Geometry: see drawing. Coordinates: mm, zero at the bounding-box minimum. Round coordinates to 2 decimals unless told otherwise and drop trailing zeros. Loops run counter-clockwise (first coordinate to the right, second up) from the corner with the lowest first, then second, coordinate; pieces in that order, holes last.
(1) Section C-C, the plane y = 1.4. Return the cut outline in (x, z).
(2) Mould query, pull axis Z, two halves, no side actions, for the marked faces 1, 2 and 3. Classes: pulls with the +Z half, pulls with the -Z half, needs draft (parallel to the pull), parting line crosses it, or undercut.
(3) Section B-B, the plane z = 26.67. Return the cut outline in (x, y), plus the area to 3 significant figures.
(4) Section D-D, the plane x = 42. Return the cut outline in (y, z), plus the area to 3 significant figures.
(5) Material intervals for probe 1 along Z at (x, y) = (26.67, 3.4); probe 2 along X at (y, z) = (2.3, 45.72); probe 3 along Z at (x, y) = (31.5, 1.6), sorted ascending.
(6) First-contact query: pin 1 Ø3 at (x, y) = (11.5, 4) entering from +Z; pin 2 Ø1.5 at (x, y) = (12.5, 3.5) entering from -Z; pin 3 Ø2.5 at (x, y) = (27, 3) entering from -Z. Flat tips, straight axial feed; report the tip coordinate or a pass-through.
(7) Section A-A, the plane x = 26.67. Return the cut outline in (y, z).
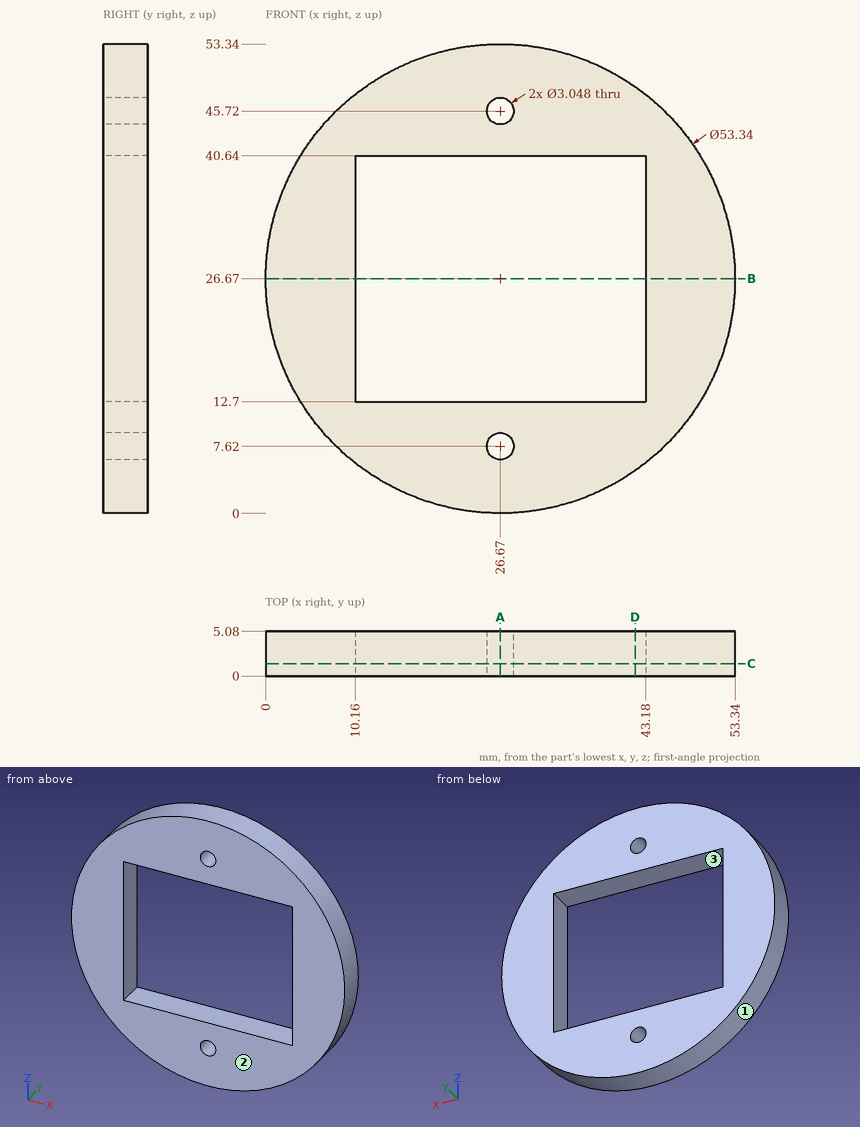
Output values:
1. outline: circle Ø53.34 at (26.67, 26.67); hole (10.16, 12.7) - (43.18, 12.7) - (43.18, 40.64) - (10.16, 40.64) - close; hole circle Ø3.05 at (26.67, 7.62); hole circle Ø3.05 at (26.67, 45.72)
2. face 1: parting line crosses it
2. face 2: needs draft
2. face 3: undercut
3. outline: (0, 0) - (10.16, 0) - (10.16, 5.08) - (0, 5.08) - close; (43.18, 0) - (53.34, 0) - (53.34, 5.08) - (43.18, 5.08) - close
3. area: 103 mm2
4. outline: (0, 4.85) - (5.08, 4.85) - (5.08, 12.7) - (0, 12.7) - close; (0, 40.64) - (5.08, 40.64) - (5.08, 48.49) - (0, 48.49) - close
4. area: 79.8 mm2
5. probe 1: z = 0 to 6.1, 9.14 to 12.7, 40.64 to 44.2, 47.24 to 53.34
5. probe 2: x = 8 to 25.15, 28.19 to 45.34
5. probe 3: z = 0.44 to 12.7, 40.64 to 52.9
6. pin 1: stops at z = 49.57
6. pin 2: stops at z = 3.62
6. pin 3: stops at z = 0
7. outline: (0, 0) - (5.08, 0) - (5.08, 6.1) - (0, 6.1) - close; (0, 9.14) - (5.08, 9.14) - (5.08, 12.7) - (0, 12.7) - close; (0, 40.64) - (5.08, 40.64) - (5.08, 44.2) - (0, 44.2) - close; (0, 47.24) - (5.08, 47.24) - (5.08, 53.34) - (0, 53.34) - close
